```python
from build123d import *

# Parameters (mm, degrees)
SKETCH1_R           = 48.895
BOSS_EXTRUDE1_DEPTH = 23.368
FILLET1_R           = 2.54
FILLET2_R           = 2.54
SKETCH2_R           = 4.225692655
CUT_EXTRUDE1_DEPTH  = 3.048


with BuildPart() as part:
    # Sketch1 → Boss-Extrude1 (new body)
    with BuildSketch(Plane.XY):
        Circle(SKETCH1_R)
    extrude(amount=BOSS_EXTRUDE1_DEPTH)

    # Fillet1
    fillet1_edges = [part.edges().sort_by_distance(p)[0] for p in [
        (-48.895, 0, 23.368),
    ]]
    fillet(fillet1_edges, radius=FILLET1_R)

    # Fillet2
    fillet2_edges = [part.edges().sort_by_distance(p)[0] for p in [
        (-48.895, 0, 0),
    ]]
    fillet(fillet2_edges, radius=FILLET2_R)

    # Sketch2 → Cut-Extrude1 (cut)
    with BuildSketch(Plane.XY.offset(23.368)):
        Circle(SKETCH2_R)
    extrude(amount=-CUT_EXTRUDE1_DEPTH, mode=Mode.SUBTRACT)


solid = part.part
```
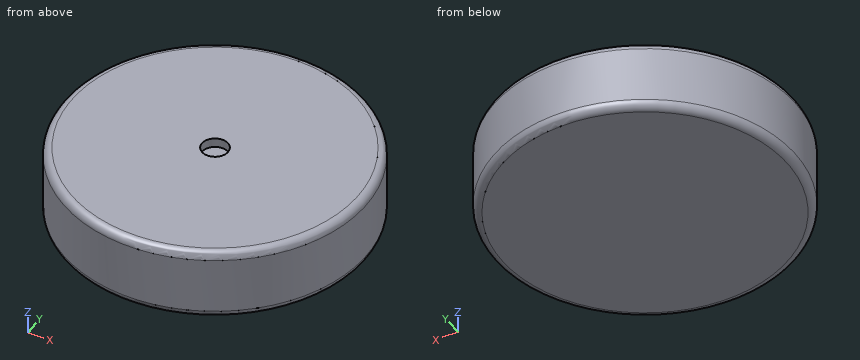
For this review, take the finished solid that the model builds, in its own axes (mm). Coordinates: 2 decimals unless noted, no trailing zeros. Write each loop counter-clockwise with the first axis right and the second up, starting at its lowest first coordinate (ties: lowest second). Pieces come first, ordered by that corner, then holes. Notation, with made-up numbers: (70.5, 50) - (92.5, 50) arc R28 ccw to (92.5, 85) - close; hole circle Ø8 at (5.25, -15). An arc over 180 degrees is marked (long way). Answer in a Markdown table with one row per item. Add a question column.
Q1. For P1, Ø10, axis at x = -35, z = 11.5, coming from the +Y side; P2, Ø12, axis at x = -25, z = 3, coming from the -Y side; P3, Ø5, axis at x = -31, z = 13, coming from the -Y side, all flat-tipped, find the tip position at first contact; note any pin that passes through.
Q2. We need section A-A, the plane z = 12.75. State the section outline as (x, y) points (3 decimals).
Q3. For probe 1 along Y at (x, z) = (0, 22.6); probe 2 along Y at (x, z) = (0, 22.4); probe 3 along Y at (x, z) = (33, 13.75), list the stretches that pass through material, from the lowest coordinate up.
Answer list:
| question | item | result |
|---|---|---|
| 1 | P1 | stops at y = 38.61 |
| 1 | P2 | stops at y = -45.05 |
| 1 | P3 | stops at y = -39.73 |
| 2 | outline | circle Ø97.79 at (0, 0) |
| 3 | probe 1 | y = -48.17 to -4.23, 4.23 to 48.17 |
| 3 | probe 2 | y = -48.35 to -4.23, 4.23 to 48.35 |
| 3 | probe 3 | y = -36.08 to 36.08 |
